Geometry: final body of the model. Coordinates: model frame, mm. Face numbers are marked on the shaded views. Round coordinates to 2 decimals unless told otherwise and drop trailing zeros. Write each loop counter-clockwise with the first axis right and the second up, starting at its lowest first coordinate (ties: lowest second). Pieces come first, ordered by that corner, then holes. Notation, with made-up numbers: (-20, -18) - (-4, -18) arc R10 ccw to (-4, 1) - close; hole circle Ø5 at (57.25, 22.25). An arc over 180 degrees is marked (long way). Write each question's results on one line, items separated by ' | '.
Autodesk Inventor part; units mm, degrees
ref_plane "YZ Plane" through (0, 0, 0) normal (1, 0, 0) x (0, 1, 0)
ref_plane "XZ Plane" through (0, 0, 0) normal (0, 1, 0) x (-1, 0, 0)
ref_plane "XY Plane" through (0, 0, 0) normal (0, 0, 1) x (1, 0, 0)
sketch "Sketch1" plane through (0, 0, 0) normal (0, 0, 1) x (1, 0, 0)
  line L0 (10.1036, 0) -> (5.0518, -8.75)
  line L1 (5.0518, -8.75) -> (-5.0518, -8.75)
  line L2 (-5.0518, -8.75) -> (-10.1036, 0)
  line L3 (-10.1036, 0) -> (-5.0518, 8.75)
  line L4 (-5.0518, 8.75) -> (5.0518, 8.75)
  line L5 (5.0518, 8.75) -> (10.1036, 0)
  circle A0 centre (0, 0) radius 5.5
  dimension "d0" = 17.5
  dimension "d1" = 11
extrude "Extrusion1" add sketch "Sketch1" along normal blind 6.5
sketch "Sketch2" plane through (0, 0, 6.5) normal (0, 0, 1) x (1, 0, 0)
  circle A0 centre (0, 0) radius 8.75
  circle A1 centre (0, 0) radius 5.65
  dimension "d4" = 17.5
  dimension "d5" = 11.3
extrude "Extrusion2" add sketch "Sketch2" along normal blind 16
sketch "Sketch3" plane through (0, 0, 22.5) normal (0, 0, 1) x (1, 0, 0)
  circle A0 centre (0, 0) radius 5.65
  line L0 (10.1036, 0) -> (5.0518, -8.75)
  line L1 (5.0518, -8.75) -> (-5.0518, -8.75)
  line L2 (-5.0518, -8.75) -> (-10.1036, 0)
  line L3 (-10.1036, 0) -> (-5.0518, 8.75)
  line L4 (-5.0518, 8.75) -> (5.0518, 8.75)
  line L5 (5.0518, 8.75) -> (10.1036, 0)
  dimension "d8" = 17.5
extrude "Extrusion3" add sketch "Sketch3" along normal blind 6
properties part number "AcopleIntermedio" material "Copper"
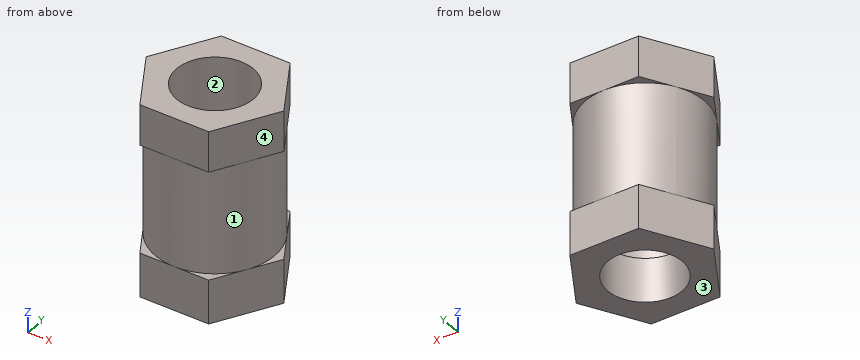
Q1. Mould query, pull axis Y, two halves, no side actions, for the marked faces 1, 2, 3 and 4. Classes: pulls with the +Y half, pulls with the -Y half, needs draft (parallel to the pull), parting line crosses it, or undercut.
Answer block:
face 1: parting line crosses it | face 2: undercut | face 3: needs draft | face 4: pulls with the -Y half
Q2. Section query A-A, the plane z = 5. Return loops of the section in (x, y), plus the area to 3 significant figures.
Answer block:
outline: (-10.1, 0) - (-5.05, -8.75) - (5.05, -8.75) - (10.1, 0) - (5.05, 8.75) - (-5.05, 8.75) - close; hole circle Ø11 at (0, 0) | area: 170 mm2
Q3. Section query C-C, the plane x = 6.5. Return loops of the section in (y, z).
Answer block:
outline: (-6.24, 0) - (6.24, 0) - (6.24, 6.5) - (5.86, 6.5) - (5.86, 22.5) - (6.24, 22.5) - (6.24, 28.5) - (-6.24, 28.5) - (-6.24, 22.5) - (-5.86, 22.5) - (-5.86, 6.5) - (-6.24, 6.5) - close
Q4. Section query B-B, the plane x = -2.25. Return loops of the section in (y, z), plus the area to 3 significant figures.
Answer block:
outline: (-8.75, 0) - (-5.02, 0) - (-5.02, 6.5) - (-5.18, 6.5) - (-5.18, 28.5) - (-8.75, 28.5) - (-8.75, 22.5) - (-8.46, 22.5) - (-8.46, 6.5) - (-8.75, 6.5) - close; (5.02, 0) - (8.75, 0) - (8.75, 6.5) - (8.46, 6.5) - (8.46, 22.5) - (8.75, 22.5) - (8.75, 28.5) - (5.18, 28.5) - (5.18, 6.5) - (5.02, 6.5) - close | area: 196 mm2
Q5. Ray query, line 1 along Y through (x, z) = (0, 20.75); line 2 along Z through (x, y) = (9, 1); line 3 along Y through (x, z) = (0, 3.75). Return the intervals inside material, ascending.
Answer block:
line 1: -8.75 to -5.65, 5.65 to 8.75 | line 2: 0 to 6.5, 22.5 to 28.5 | line 3: -8.75 to -5.5, 5.5 to 8.75
Q6. Section query D-D, the plane y = -7. Return loops of the section in (x, z), plus the area to 3 significant figures.
Answer block:
outline: (-6.06, 0) - (6.06, 0) - (6.06, 6.5) - (5.25, 6.5) - (5.25, 22.5) - (6.06, 22.5) - (6.06, 28.5) - (-6.06, 28.5) - (-6.06, 22.5) - (-5.25, 22.5) - (-5.25, 6.5) - (-6.06, 6.5) - close | area: 320 mm2
Q7. Pin query (flat end, axial travel): pin 1 (2 mm diameter, centred on x = 5, z = 8, fed in from -Y); pin 2 (6 mm diameter, centred on y = 2, z = 13.5, fed in from -X); pin 3 (5 mm diameter, centred on x = 5, z = 17.5, fed in from +Y). Return the tip coordinate at first contact, or that it passes through.
Answer block:
pin 1: y = -7.78 | pin 2: x = -8.75 | pin 3: y = 8.39
